```python
from build123d import *

# Parameters (mm, degrees)
SKETCH1_R           = 1.55
SKETCH1_R_2         = 2
BOSS_EXTRUDE1_DEPTH = 2.5
CUT_EXTRUDE1_START  = -2
CUT_EXTRUDE1_DEPTH  = 2
FILLET1_R           = 2


with BuildPart() as part:
    # Sketch1 → Boss-Extrude1 (new, symmetric)
    with BuildSketch(Plane.XY):
        with BuildLine():
            Line((-8.93028555, 4.5), (30, 4.5))
            ThreePointArc((30, 4.5), (34.5, 0), (30, -4.5))
            Line((30, -4.5), (-8.93028555, -4.5))
            ThreePointArc((-8.93028555, -4.5), (-10, 0), (-8.93028555, 4.5))
        make_face()
        with Locations((-7, 0)):
            Circle(SKETCH1_R, mode=Mode.SUBTRACT)
        with Locations((7, 0)):
            Circle(SKETCH1_R, mode=Mode.SUBTRACT)
        with Locations((30, 0)):
            Circle(SKETCH1_R, mode=Mode.SUBTRACT)
        Circle(SKETCH1_R_2, mode=Mode.SUBTRACT)
    extrude(amount=BOSS_EXTRUDE1_DEPTH, both=True)

    # Sketch2 → Cut-Extrude1 (cut)
    with BuildSketch(Plane(origin=(0, 0, -2.5), x_dir=(-1, 0, 0), z_dir=(0, 0, -1)).offset(CUT_EXTRUDE1_START)):
        with BuildLine():
            Line((-30, 4.5), (-8.93028555, 4.5))
            ThreePointArc((-8.93028555, 4.5), (-10, 0), (-8.93028555, -4.5))
            Line((-8.93028555, -4.5), (-30, -4.5))
            ThreePointArc((-30, -4.5), (-34.5, 0), (-30, 4.5))
        make_face()
    extrude(amount=CUT_EXTRUDE1_DEPTH, mode=Mode.SUBTRACT)

    # Fillet1
    fillet1_edges = [part.edges().sort_by_distance(p)[0] for p in [
        (8.93028555, 4.5, -1.5),
        (8.93028555, -4.5, -1.5),
        (-8.93028555, 4.5, 0),
        (-8.93028555, -4.5, 0),
    ]]
    fillet(fillet1_edges, radius=FILLET1_R)


solid = part.part
```
The model under review builds one solid part; all positions refer to its coordinate system, in mm. A direction names the side the tool comes from. Coordinates: 2 decimals unless noted, no trailing zeros. Write each loop counter-clockwise with the first axis right and the second up, starting at its lowest first coordinate (ties: lowest second). Pieces come first, ordered by that corner, then holes. Notation, with made-up numbers: (18.5, -27) - (60.5, -27) arc R16 ccw to (60.5, -2) - close; hole circle Ø8 at (79, 34). An arc over 180 degrees is marked (long way). Answer in a Markdown table with one row per item. Add a question column.
Q1. Clearance check with flat-ended pins moving along their axes: pin 1 (3 mm diameter, centred on y = -2, z = 1, fed in from +X); pin 2 (3 mm diameter, centred on x = 30, y = 1, fed in from -Z). State where each tip first meets the part, or that it passes through.
Q2. For faces 1 (the face through (8.8, 4.1, -1.5)), 2 (the face through (7, -4.5, 1)), 3 (the face through (10, 0, -1)), list the 3-axis set-ups (+Z, -Z, +X, -X, +Y, -Y) from which the entire face can be reached by the end or side of a thin tool; tool diameter is ignored.
Q3. Consider section C-C on x = 0. Give the boundary of the cut face in (y, z).
Q4. Consider section D-D on x = 7. Give the boundary of the cut face in (y, z), then the cut area to 3 significant figures.
Q5. Consider section A-A on z = -1. Give the boundary of the cut face in (x, y) (3 decimals), then the cut area to 3 significant figures.
Q6. To check wall thickness, follow line 1 along Y through (x, z) = (7, -0.05); line 2 along Y through (x, z) = (0, 0); line 3 along X through (y, z) = (0.5, -1.95). State the ranges of each line that lie inside material, in increasing order. Write a range as from..to.
Q7. Draft analysis for pull direction Y (two halves, no side actions). For faces 4 (the face through (7, 4.5, 1)), 5 (the face through (8.8, -4.1, -1.5)), 6 (the face through (-5.522, 0.466, -0.035)), state which applies: +Y half, -Y half, draft (parallel to the pull), parting line (faces both ways), or undercut.
Q8. Consider section B-B on y = 0. Give the boundary of the cut face in (x, z), then the cut area to 3 significant figures.
Answers below:
| question | item | result |
|---|---|---|
| 1 | pin 1 | x = 34.47 |
| 1 | pin 2 | z = -0.5 |
| 2 | face 1 | -Z, +X, +Y |
| 2 | face 2 | +Z, -Z, +X, -X, -Y |
| 2 | face 3 | -Z, +X |
| 3 | outline | (-4.5, -2.5) - (-2, -2.5) - (-2, 2.5) - (-4.5, 2.5) - close; (2, -2.5) - (4.5, -2.5) - (4.5, 2.5) - (2, 2.5) - close |
| 4 | outline | (-4.5, -2.5) - (-1.55, -2.5) - (-1.55, 2.5) - (-4.5, 2.5) - close; (1.55, -2.5) - (4.5, -2.5) - (4.5, 2.5) - (1.55, 2.5) - close |
| 4 | area | 29.5 mm² |
| 5 | outline | (-9.499, -3.125) arc R2 ccw to (-7.599, -4.5) - (7.599, -4.5) arc R2 ccw to (9.499, -3.125) arc R10 ccw to (9.499, 3.125) arc R2 ccw to (7.599, 4.5) - (-7.599, 4.5) arc R2 ccw to (-9.499, 3.125) arc R10 ccw to start; hole circle Ø3.1 at (-7, 0); hole circle Ø4 at (0, 0); hole circle Ø3.1 at (7, 0) |
| 5 | area | 145 mm² |
| 6 | line 1 | -4.5..-1.55, 1.55..4.5 |
| 6 | line 2 | -4.5..-2, 2..4.5 |
| 6 | line 3 | -9.99..-8.47, -5.53..-1.94, 1.94..5.53, 8.47..9.99 |
| 7 | face 4 | +Y half |
| 7 | face 5 | -Y half |
| 7 | face 6 | undercut |
| 8 | outline | (-10, -2.5) - (-8.55, -2.5) - (-8.55, 2.5) - (-10, 2.5) - close; (-5.45, -2.5) - (-2, -2.5) - (-2, 2.5) - (-5.45, 2.5) - close; (2, -2.5) - (5.45, -2.5) - (5.45, 2.5) - (2, 2.5) - close; (8.55, -2.5) - (10, -2.5) - (10, -0.5) - (28.45, -0.5) - (28.45, 2.5) - (8.55, 2.5) - close; (31.55, -0.5) - (34.5, -0.5) - (34.5, 2.5) - (31.55, 2.5) - close |
| 8 | area | 113 mm² |
